Read the model definition and answer for the solid it produces. Units are mm, in the model's axes. A direction names the side the tool comes from. Round coordinates to 2 decimals unless told otherwise and drop trailing zeros. Order: outer loops, then holes, each group sorted by start corner. A loop starts at its lowest first (then second) coordinate and runs counter-clockwise, first axis right, second up. Notation, with made-up numbers: (46, -21.5) - (99, -21.5) arc R33 ccw to (99, 17.5) - close; hole circle Ø2 at (3.5, 27). An arc over 180 degrees is marked (long way). Answer as a JSON object with one key per item and string values. Group by question number.
Q1. A cutting plane is placed at D-D on y = 10.6. Determine the outline of the cut face in (x, z).
Q2. The mould has two halves that part along X. Classify faces 1 (the cylindrical face through (-3.07, 5.45, 2.54)), 2 (the flat face through (0, 1, 0)), 3 (the flat face through (-15, 0, 2)): pulls with the +X half, pulls with the -X half, needs draft (parallel to the pull), parting line crosses it, or undercut.
Q3. Consider line 1 (X direction, y = 0, z = 1.8); line 2 (Y direction, x = -5.05, z = 2.5); line 3 (Z direction, x = 5.2, y = 10.6). Determine where each line is inside the solid, lowest interval first.
Q4. Given pin 1 Ø3 at (x, z) = (-11, 2.5) entering from +Y; pin 2 Ø3 at (x, z) = (12.5, 2) entering from +Y; pin 3 Ø1.5 at (y, z) = (9, 1.5) entering from +X, each flat-ended and moving along its own axis, determine where each tip first touches the part or whether it passes through.
Q5. A tool of negligible diameter and unlimited length cuts with its end or side. For faces 4 (the cylindrical face through (-6.035, 12.552, 2.934)), 5 (the flat face through (12, 5, 2)), 6 (the cylindrical face through (3.05, 5.43, 2.54)), 7 (the flat face through (-8.5, 8, 2)), from which of +Z, -Z, +X, -X, +Y, -Y can it reach the whole face along a straight path? Write none if from no direction.
Q6. A cutting plane is placed at B-B on y = 0. Determine the outline of the cut face in (x, z).
Q7. A cutting plane is placed at A-A on z = 2.5. Count the separate pieces of the cut face and the enclosed holes in it, and give its area (3 significant figures).
Q8. A cutting plane is placed at C-C on x = -6. Determine the outline of the cut face in (y, z).
Autodesk Inventor part; units mm, degrees
ref_plane "YZ Plane" through (0, 0, 0) normal (1, 0, 0) x (0, 1, 0)
ref_plane "XZ Plane" through (0, 0, 0) normal (0, 1, 0) x (-1, 0, 0)
ref_plane "XY Plane" through (0, 0, 0) normal (0, 0, 1) x (1, 0, 0)
sketch "Sketch1" plane through (0, 0, 0) normal (0, 0, 1) x (1, 0, 0)
  line L0 (-15, -5) -> (15, -5)
  line L1 (15, -5) -> (15, 5)
  line L2 (15, 5) -> (-15, 5)
  line L3 (-15, 5) -> (-15, -5)
  line L4 (-15, -5) -> (15, 5) construction
  line L5 (15, -5) -> (-15, 5) construction
  line L6 (-8.5, 5) -> (-8.5, 13)
  line L7 (-8.5, 13) -> (-3.5, 13)
  line L8 (-3.5, 13) -> (-3.5, 5)
  line L9 (0, 0) -> (0, 10.7683) construction
  line L10 (8.5, 5) -> (8.5, 13)
  line L11 (8.5, 13) -> (3.5, 13)
  line L12 (3.5, 13) -> (3.5, 5)
  point P0 (8.5, 5)
  point P1 (3.5, 5)
  dimension "d0" = 10
  dimension "d1" = 30
  dimension "d2" = 5
  dimension "d3" = 8
  dimension "d4" = 7
extrude "Extrusion1" add sketch "Sketch1" along normal blind 5
sketch "Sketch2" plane through (8.5, 5, 0) normal (1, 0, 0) x (0, 0, -1)
  line L0 (0, 0) -> (0, 8)
  line L1 (-5, 0) -> (-5, 8)
  line L2 (0, 8) -> (-5, 8)
  line L3 (0, 0) -> (-5, 0)
  point P0 (0, -5)
  point P1 (-2.5, 5.6)
  dimension "d14" = 2.5
  dimension "d15" = 5
  dimension "d16" = 2.4
  dimension "d17" = 8
hole "Hole1" at (8.5, 10.6, 2.5) direction (-1, 0, 0) diameter 4 end through all
fillet "Fillet1" radius 2 4 edges at (6, 13, 0) (6, 13, 5) (-6, 13, 0) (-6, 13, 5)
fillet "Fillet2" radius 1.5 8 edges at (-3.5, 5, 2.5) (3.5, 5, 2.5) (-8.5, 5, 2.5) (8.5, 5, 2.5) (15, 5, 2.5) (15, -5, 2.5) (-15, -5, 2.5) (-15, 5, 2.5)
sketch "Sketch3" plane through (0, 0, 5) normal (0, 0, 1) x (1, 0, 0)
  point P0 (0, 0)
  point P1 (-10, 0)
  point P2 (10, 0)
  dimension "d27" = 10
  dimension "d30" = 360
hole "Hole2" at (-10, 0, 5) at (10, 0, 5) direction (0, 0, -1) diameter 5.5 end through all
properties part number "axe_camera"
Result set:
{
 "1": {"outline": "(-8.5, 0) - (-3.5, 0) - (-3.5, 0.5) - (-8.5, 0.5) - close; (-8.5, 4.5) - (-3.5, 4.5) - (-3.5, 5) - (-8.5, 5) - close; (3.5, 0) - (8.5, 0) - (8.5, 0.5) - (3.5, 0.5) - close; (3.5, 4.5) - (8.5, 4.5) - (8.5, 5) - (3.5, 5) - close"},
 "2": {"face 1": "undercut", "face 2": "needs draft", "face 3": "pulls with the -X half"},
 "3": {"line 1": "x = -15 to -12.75, -7.25 to 7.25, 12.75 to 15", "line 2": "y = -5 to 8.6, 12.6 to 13", "line 3": "z = 0 to 0.5, 4.5 to 5"},
 "4": {"pin 1": "stops at y = 5.09", "pin 2": "stops at y = 5", "pin 3": "stops at x = 8.5"},
 "5": {"face 4": "+X, -X", "face 5": "+Z, -Z, +X, +Y", "face 6": "+Z, -Z, +Y", "face 7": "+Z, -Z, -X, +Y"},
 "6": {"outline": "(-15, 0) - (-12.75, 0) - (-12.75, 5) - (-15, 5) - close; (-7.25, 0) - (7.25, 0) - (7.25, 5) - (-7.25, 5) - close; (12.75, 0) - (15, 0) - (15, 5) - (12.75, 5) - close"},
 "7": {"separate pieces": "3", "enclosed holes": "2", "area": "292 mm²"},
 "8": {"outline": "(-5, 0) - (11, 0) arc R2 ccw to (13, 2) - (13, 3) arc R2 ccw to (11, 5) - (-5, 5) - close; hole circle Ø4 at (10.6, 2.5)"}
}
